```python
from build123d import *

# Parameters (mm, degrees)
BOSS_EXTRUDE1_DEPTH = 1.32
FILLET1_R           = 3
FILLET2_R           = 1.6


with BuildPart() as part:
    # Sketch1 → Boss-Extrude1 (new body)
    with BuildSketch(Plane(origin=(0, 0, 0), x_dir=(1, 0, 0), z_dir=(0, 1, 0))):
        Polygon((0, 4.51), (0, 0), (23.8, 0), (23.8, 12.82), (4.6, 12.82), (4.6, 4.51), align=None)
    extrude(amount=BOSS_EXTRUDE1_DEPTH)

    # Fillet1
    fillet1_edges = [part.edges().sort_by_distance(p)[0] for p in [
        (4.6, 0.66, -12.82),
        (23.8, 0.66, 0),
    ]]
    fillet(fillet1_edges, radius=FILLET1_R)

    # Fillet2
    fillet2_edges = [part.edges().sort_by_distance(p)[0] for p in [
        (0, 0.66, -4.51),
        (4.6, 0.66, -4.51),
        (23.8, 0.66, -12.82),
        (0, 0.66, 0),
    ]]
    fillet(fillet2_edges, radius=FILLET2_R)


solid = part.part
```
CAD build for the part. Positions are in the model's coordinates, mm. A direction names the side the tool comes from. Coordinates: 2 decimals unless noted, no trailing zeros. Write each loop counter-clockwise with the first axis right and the second up, starting at its lowest first coordinate (ties: lowest second). Pieces come first, ordered by that corner, then holes.
(1) Cut at A-A, the plane y = 0.7. List the corners of the cut face in (x, z).
(2) Cut at C-C, the plane x = 2. List the corners of the cut face in (y, z).
(3) Drill centre lines: probe 1 along X at (y, z) = (1, -7.25); probe 2 along Z at (x, y) = (1.5, 0.75); probe 3 along X at (y, z) = (0.95, -1.5). Where is each one in solid material? Low to high.
(4) 3-axis set-ups, long thin cutter, end or side, ignore diameter. For faces 1 (the face through (4.6, 1, -8)), 2 (the face through (15, 1, -12.82)): which of +Z, -Z, +X, -X, +Y, -Y reach the whole face in a straight line?
(5) Cut at B-B, the plane z = -7.75. List the corners of the cut face in (x, y).
Geometry says:
1. outline: (0, -2.91) arc R1.6 ccw to (1.6, -4.51) - (3, -4.51) arc R1.6 cw to (4.6, -6.11) - (4.6, -9.82) arc R3 ccw to (7.6, -12.82) - (22.2, -12.82) arc R1.6 ccw to (23.8, -11.22) - (23.8, -3) arc R3 ccw to (20.8, 0) - (1.6, 0) arc R1.6 ccw to (0, -1.6) - close
2. outline: (0, -4.51) - (1.32, -4.51) - (1.32, 0) - (0, 0) - close
3. probe 1: x = 4.6 to 23.8
3. probe 2: z = -4.51 to 0
3. probe 3: x = 0 to 23.4
4. face 1: -Z, -X, +Y, -Y
4. face 2: -Z, +X, -X, +Y, -Y
5. outline: (4.6, 0) - (23.8, 0) - (23.8, 1.32) - (4.6, 1.32) - close
